Check sheet for the modelled part. Datum: model origin and axes. Units: mm. Face numbers are marked on the shaded views. A direction names the side the tool comes from. Round coordinates to 2 decimals unless told otherwise and drop trailing zeros. Write each loop counter-clockwise with the first axis right and the second up, starting at its lowest first coordinate (ties: lowest second). Pieces come first, ordered by that corner, then holes.
Item 1: Cross-section at D-D on z = 23.5. Enter the section's corners in (x, y).
Item 2: Material ranges on line 1 (Z direction, x = -1.45, y = -10); line 2 (Z direction, x = 17.5, y = -39.5); line 3 (Y direction, x = 30.5, z = 18.5), recorded low to high.
Item 3: Go/stop test with flat-tipped pins: pin 1 Ø3.5 at (y, z) = (-10, 17.5) entering from +X; pin 2 Ø5 at (y, z) = (-18, 10.5) entering from +X; pin 3 Ø10 at (x, z) = (18.5, 13.5) entering from +Y. Record where each tip stops, or that it passes through.
Item 4: Cross-section at A-A on z = 17.5. Enter the section's corners in (x, y).
Item 5: Tool access check on the marked faces 1 and 2. Record the directions out of +Z, -Z, +X, -X, +Y, -Y that give a thin tool (end or side, any length) a straight path to the whole face; none if there is none.
Item 6: Cross-section at C-C on x = 17.5. Enter the section's corners in (y, z).
Item 7: Cross-section at B-B on y = -10. Enter the section's corners in (x, z).
from build123d import *

# Parameters (mm, degrees)
BOSS_EXTRU_1_DEPTH      = 35
ESQUISSE2_R             = 8
ENL_V_MAT_EXTRU_1_DEPTH = 20
ESQUISSE3_R             = 3
ENL_V_MAT_EXTRU_2_DEPTH = 20
CONG_1_R                = 10


with BuildPart() as part:
    # Esquisse1 → Boss.-Extru.1 (new body)
    with BuildSketch(Plane.XY):
        Polygon((0, 0), (0, -37.5), (32.5, -37.5), (32.5, -40), (-2.5, -40), (-2.5, 0), align=None)
    extrude(amount=BOSS_EXTRU_1_DEPTH)

    # Esquisse2 → Enlèv. mat.-Extru.1 (cut)
    with BuildSketch(Plane(origin=(0, -40, 0), x_dir=(-1, 0, 0), z_dir=(0, -1, 0))):
        with Locations(Location((-17.5, -17.5, 0), (0, 0, 180))):
            Circle(ESQUISSE2_R)
    extrude(amount=-ENL_V_MAT_EXTRU_1_DEPTH, mode=Mode.SUBTRACT)

    # Esquisse3 → Enlèv. mat.-Extru.2 (cut)
    with BuildSketch(Plane(origin=(0, 0, 0), x_dir=(0, 0, -1), z_dir=(1, 0, 0))):
        with Locations(Location((-17.5, -10, 0), (0, 0, 90))):
            Circle(ESQUISSE3_R)
        with Locations(Location((-17.5, -30, 0), (0, 0, 90))):
            Circle(ESQUISSE3_R)
    extrude(amount=-ENL_V_MAT_EXTRU_2_DEPTH, mode=Mode.SUBTRACT)

    # Congé1
    cong_1_edges = [part.edges().sort_by_distance(p)[0] for p in [
        (32.5, -38.75, 35),
        (32.5, -38.75, 0),
    ]]
    fillet(cong_1_edges, radius=CONG_1_R)


solid = part.part
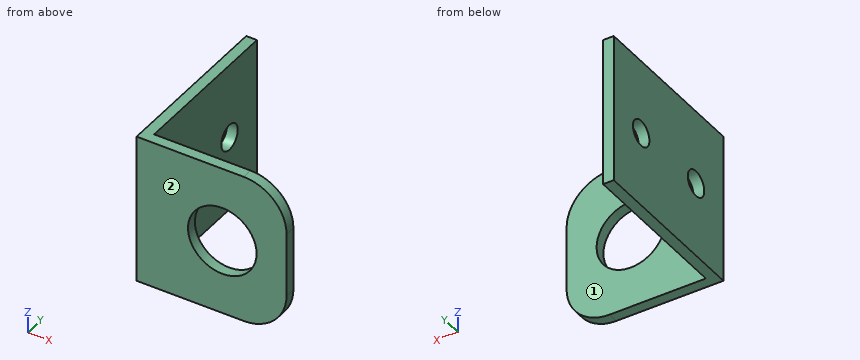
Response values:
1. outline: (-2.5, -40) - (12.21, -40) - (12.21, -37.5) - (0, -37.5) - (0, 0) - (-2.5, 0) - close; (22.79, -40) - (32.5, -40) - (32.5, -37.5) - (22.79, -37.5) - close
2. line 1: z = 0 to 14.5, 20.5 to 35
2. line 2: z = 0 to 9.5, 25.5 to 35
2. line 3: y = -40 to -37.5
3. pin 1: passes through
3. pin 2: stops at x = 0
3. pin 3: stops at y = -37.5
4. outline: (-2.5, -40) - (9.5, -40) - (9.5, -37.5) - (0, -37.5) - (0, -33) - (-2.5, -33) - close; (-2.5, -27) - (0, -27) - (0, -13) - (-2.5, -13) - close; (-2.5, -7) - (0, -7) - (0, 0) - (-2.5, 0) - close; (25.5, -40) - (32.5, -40) - (32.5, -37.5) - (25.5, -37.5) - close
5. face 1: +Z, -Z, +X, +Y
5. face 2: +Z, -Z, +X, -X, -Y
6. outline: (-40, 0) - (-37.5, 0) - (-37.5, 9.5) - (-40, 9.5) - close; (-40, 25.5) - (-37.5, 25.5) - (-37.5, 35) - (-40, 35) - close
7. outline: (-2.5, 0) - (0, 0) - (0, 14.5) - (-2.5, 14.5) - close; (-2.5, 20.5) - (0, 20.5) - (0, 35) - (-2.5, 35) - close
